from build123d import *

# Parameters (mm, degrees)
SKETCH1_W           = 300
SKETCH1_H           = 300
BOSS_EXTRUDE1_DEPTH = 40
SKETCH2_W           = 20
SKETCH2_H           = 20
BOSS_EXTRUDE2_DEPTH = 200


with BuildPart() as part:
    # Sketch1 → Boss-Extrude1 (new body)
    with BuildSketch(Plane.XY):
        Rectangle(SKETCH1_W, SKETCH1_H)
    extrude(amount=BOSS_EXTRUDE1_DEPTH)

    # Sketch2 → Boss-Extrude2 (add)
    with BuildSketch(Plane.XY.offset(40)):
        with Locations((110, 110)):
            Rectangle(SKETCH2_W, SKETCH2_H)
        with Locations((-110, 110)):
            Rectangle(SKETCH2_W, SKETCH2_H)
        with Locations((-110, -110)):
            Rectangle(SKETCH2_W, SKETCH2_H)
        with Locations((110, -110)):
            Rectangle(SKETCH2_W, SKETCH2_H)
    extrude(amount=BOSS_EXTRUDE2_DEPTH)


solid = part.part
Source: CAD feature listing. Evaluate the final solid. Frame: model axes, mm. A direction names the side the tool comes from. Give positions to 0.01 mm unless a question says otherwise; leave off trailing zeros. Write each loop counter-clockwise with the first axis right and the second up, starting at its lowest first coordinate (ties: lowest second). Pieces come first, ordered by that corner, then holes. Notation, with made-up numbers: (15, -23) -> (44, -23) arc R17 ccw to (44, 10) -> close; hole circle Ø3 at (18.25, -22). An arc over 180 degrees is marked (long way). Return JSON: item names as keys, results as strings. Group by question number.
1. Mould query, pull axis X, two halves, no side actions, for faces 4 (the face through (-2, 150, 20)), 5 (the face through (100, -110, 139)), 6 (the face through (-120, -110, 139)). Classes: +X half, -X half, draft (parallel to the pull), parting line (faces both ways), or undercut.
2. Material intervals for line 1 (Y direction, x = -113, z = 123); line 2 (Z direction, x = 97, y = -49), sorted ascending. Write a range as from..to.
3. Pin query (flat end, axial travel): pin 1 Ø6 at (y, z) = (-112.5, 93.5) entering from +X; pin 2 Ø10 at (y, z) = (-108.5, 185.5) entering from -X; pin 3 Ø2 at (x, y) = (-37.5, 108.5) entering from +Z. Return the tip coordinate at first contact, or that it passes through.
4. Section B-B, the plane x = 105.5. Output: boundary loops of the cut face in (y, z), then the cut area to 3 significant figures.
5. Section A-A, the plane z = 161. Output: boundary loops of the cut face in (x, y), then the cut area to 3 significant figures.
6. Section C-C, the plane y = 82.5. Output: boundary loops of the cut face in (x, z).
7. Access query for faces 1 (the face through (100, 110, 139)), 2 (the face through (110, -100, 139)), 3 (the face through (110, 120, 139)). Directions: +Z, -Z, +X, -X, +Y, -Y. A direction counts if a zero-diameter tool reaches every point of the face in a straight line with its end or side. Return the directions, or none.
Determined:
{
 "1": {"face 4": "draft", "face 5": "undercut", "face 6": "-X half"},
 "2": {"line 1": "y = -120..-100, 100..120", "line 2": "z = 0..40"},
 "3": {"pin 1": "stops at x = 120", "pin 2": "stops at x = -120", "pin 3": "stops at z = 40"},
 "4": {"outline": "(-150, 0) -> (150, 0) -> (150, 40) -> (120, 40) -> (120, 240) -> (100, 240) -> (100, 40) -> (-100, 40) -> (-100, 240) -> (-120, 240) -> (-120, 40) -> (-150, 40) -> close", "area": "20,000 mm2"},
 "5": {"outline": "(-120, -120) -> (-100, -120) -> (-100, -100) -> (-120, -100) -> close; (-120, 100) -> (-100, 100) -> (-100, 120) -> (-120, 120) -> close; (100, -120) -> (120, -120) -> (120, -100) -> (100, -100) -> close; (100, 100) -> (120, 100) -> (120, 120) -> (100, 120) -> close", "area": "1,600 mm2"},
 "6": {"outline": "(-150, 0) -> (150, 0) -> (150, 40) -> (-150, 40) -> close"},
 "7": {"face 1": "+Z, +Y, -Y", "face 2": "+Z, +X, -X", "face 3": "+Z, +X, -X, +Y"}
}
